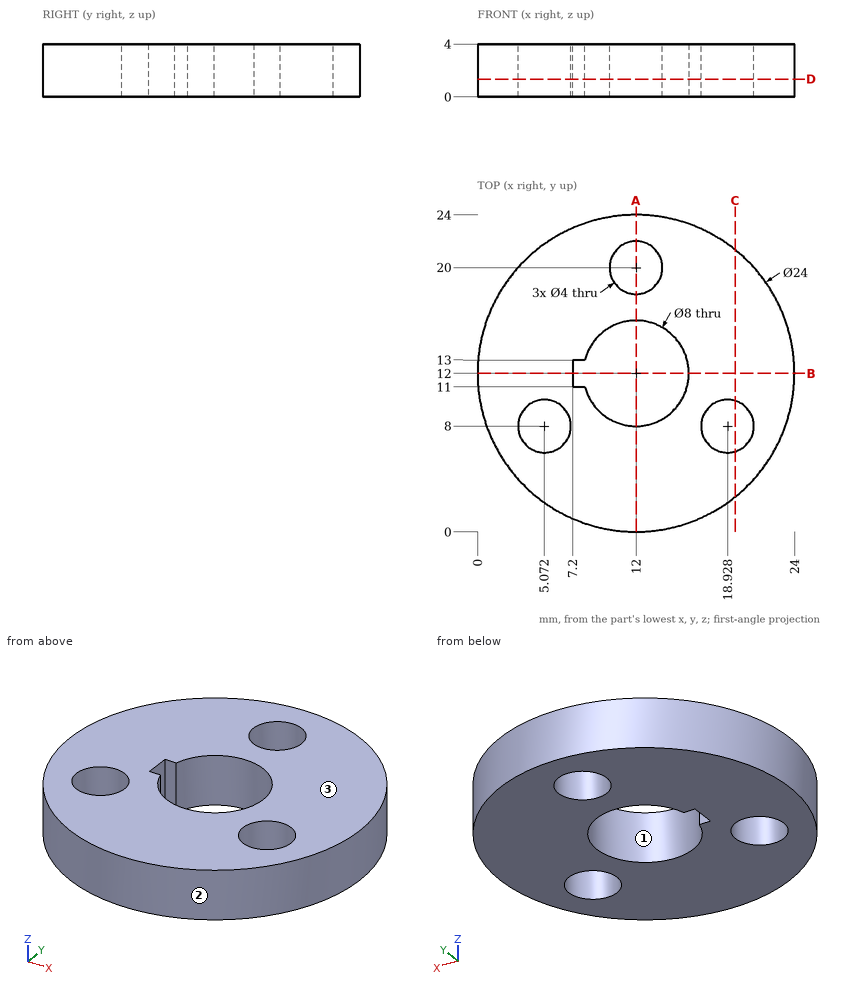
Design review of the part shown in the three views and the two pictorial views. Dimensions are in mm from the part's minimum x, y and z. Round coordinates to 2 decimals unless told otherwise and drop trailing zeros. Loops run counter-clockwise (first coordinate to the right, second up) from the corner with the lowest first, then second, coordinate; pieces in that order, holes last.
(1) We need section D-D (z = 1.35). Give the boundary of the cut face in (x, y), plus the area to 3 significant figures.
Returned:
outline: circle Ø24 at (12, 12); hole circle Ø4 at (5.07, 8); hole (7.2, 11) - (8.13, 11) arc R4 ccw (long way) to (8.13, 13) - (7.2, 13) - close; hole circle Ø4 at (12, 20); hole circle Ø4 at (18.93, 8)
area: 363 mm2
(2) We need section C-C (x = 19.5). Give the boundary of the cut face in (y, z), plus the area to 3 significant figures.
Returned:
outline: (2.63, 0) - (6.08, 0) - (6.08, 4) - (2.63, 4) - close; (9.92, 0) - (21.37, 0) - (21.37, 4) - (9.92, 4) - close
area: 59.6 mm2
(3) We need section B-B (y = 12). Give the boundary of the cut face in (x, z), plus the area to 3 significant figures.
Returned:
outline: (0, 0) - (7.2, 0) - (7.2, 4) - (0, 4) - close; (16, 0) - (24, 0) - (24, 4) - (16, 4) - close
area: 60.8 mm2
(4) Wall thickness on line 1 along Y through (x, z) = (12, 2.7); line 2 along Y through (x, z) = (11, 3.15); line 3 along X through (y, z) = (7, 1.7): over which ranges is each line inside the solid? List them lowest first.
Returned:
line 1: y = 0 to 8, 16 to 18, 22 to 24
line 2: y = 0.04 to 8.13, 15.87 to 18.27, 21.73 to 23.96
line 3: x = 1.09 to 3.34, 6.8 to 17.2, 20.66 to 22.91
(5) Clearance check with flat-ended pins moving along their axes: P1, Ø0.7, axis at x = 7.5, z = 3, coming from the +Y side; P2, Ø9, axis at x = 12, y = 12, coming from the -Z side; P3, Ø2, axis at x = 18, z = 2, coming from the -Y side; P4, Ø0.7, axis at x = 7.5, z = 2, coming from the -Y side. State where each tip first meets the part, or that it passes through.
Returned:
P1: stops at y = 23.26
P2: stops at z = 0
P3: stops at y = 1.09
P4: stops at y = 0.74
(6) Mouldability with a two-part tool opening along Y and no side actions: class the marked faces 1, 2 and 3 as released by +Y, released by -Y, zero draft, split by the parting line, or undercut.
Returned:
face 1: undercut
face 2: split by the parting line
face 3: zero draft
(7) We need section A-A (x = 12). Give the boundary of the cut face in (y, z), plus the area to 3 significant figures.
Returned:
outline: (0, 0) - (8, 0) - (8, 4) - (0, 4) - close; (16, 0) - (18, 0) - (18, 4) - (16, 4) - close; (22, 0) - (24, 0) - (24, 4) - (22, 4) - close
area: 48.0 mm2
